Design review of the part shown in the three views and the two pictorial views. Dimensions are in mm from the part's minimum x, y and z. Round coordinates to 2 decimals unless told otherwise and drop trailing zeros. Loops run counter-clockwise (first coordinate to the right, second up) from the corner with the lowest first, then second, coordinate; pieces in that order, holes last. Notation, with made-up numbers: (-19, 82) -> (-2, 82) arc R10 cw to (-2, 99) -> close; hole circle Ø8 at (-15, 37.5). An arc over 180 degrees is marked (long way). Use a Markdown table: item, result. Add a question column.
1) Consider section B-B on x = 15. Give the boundary of the cut face in (y, z).
2) Consider section C-C on z = 3.8. State how many separate pieces and enclosed holes the cut face has, plus the area to 3 significant figures.
3) Wall thickness on probe 1 along X at (y, z) = (95, 2.75); probe 2 along Y at (x, z) = (7.5, 0.25): over which ranges is each line inside the solid? List them lowest first.
4) Insertion check: pin 1 (1.5 mm diameter, centred on x = 53, z = 2.5, fed in from +Y); pin 2 (1.5 mm diameter, centred on x = 52, z = 3.5, fed in from -Y); pin 3 (3 mm diameter, centred on x = 34.5, z = 3.5, fed in from -Y). Each pin has a flat end and moves straight along its axis. Give the tip position at first contact, or say it passes through.
5) Mouldability with a two-part tool opening along Z and no side actions: class the marked faces 1 and 2 as released by +Z, released by -Z, zero draft, split by the parting line, or undercut.
6) Consider section A-A on y = 250.5. Give the boundary of the cut face in (x, z), plus the area to 3 significant figures.
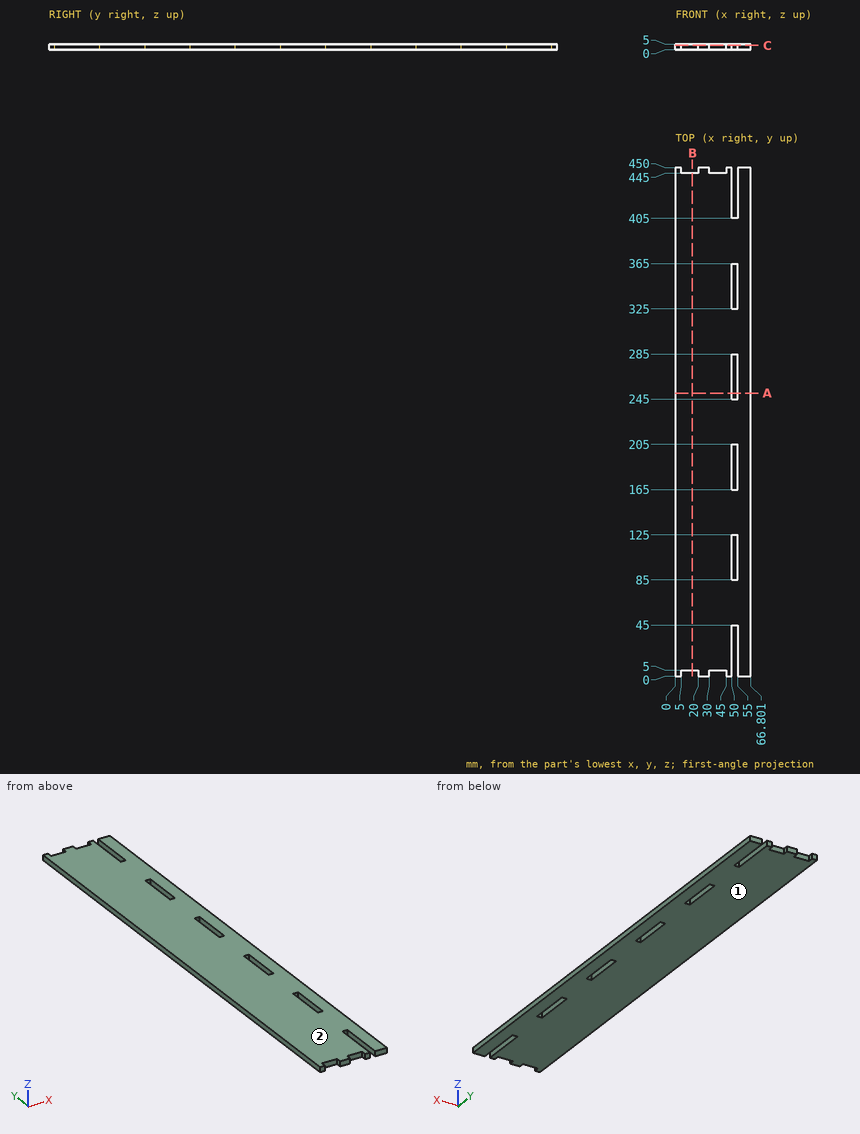
Result set:
| question | item | result |
|---|---|---|
| 1 | outline | (5, 0) -> (445, 0) -> (445, 5) -> (5, 5) -> close |
| 2 | separate pieces | 1 |
| 2 | enclosed holes | 4 |
| 2 | area | 28,500 mm2 |
| 3 | probe 1 | 0 to 50, 55 to 66.8 |
| 3 | probe 2 | 5 to 445 |
| 4 | pin 1 | y = 405 |
| 4 | pin 2 | y = 45 |
| 4 | pin 3 | y = 5 |
| 5 | face 1 | released by -Z |
| 5 | face 2 | released by +Z |
| 6 | outline | (0, 0) -> (50, 0) -> (50, 5) -> (0, 5) -> close; (55, 0) -> (66.8, 0) -> (66.8, 5) -> (55, 5) -> close |
| 6 | area | 309 mm2 |
